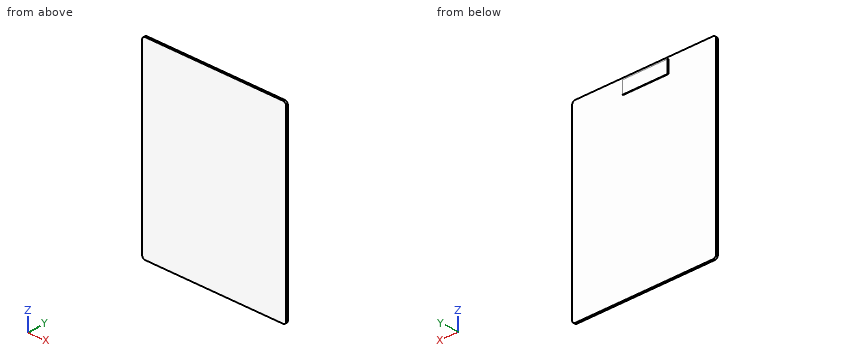
```python
from build123d import *

# Parameters (mm, degrees)
SKETCH1_W           = 230
SKETCH1_H           = 300
BOSS_EXTRUDE1_DEPTH = 3
FILLET1_R           = 5
SKETCH2_W           = 72.53015036
SKETCH2_H           = 20.073618637
BOSS_EXTRUDE2_DEPTH = 1


with BuildPart() as part:
    # Sketch1 → Boss-Extrude1 (new body)
    with BuildSketch(Plane(origin=(0, 0, 0), x_dir=(1, 0, 0), z_dir=(0, 1, 0))):
        with Locations((439.297793407, 824.401400972)):
            Rectangle(SKETCH1_W, SKETCH1_H)
    extrude(amount=BOSS_EXTRUDE1_DEPTH)

    # Fillet1
    fillet1_edges = [part.edges().sort_by_distance(p)[0] for p in [
        (554.297793407, 1.5, -674.401400972),
        (324.297793407, 1.5, -674.401400972),
        (324.297793407, 1.5, -974.401400972),
        (554.297793407, 1.5, -974.401400972),
    ]]
    fillet(fillet1_edges, radius=FILLET1_R)

    # Sketch2 → Boss-Extrude2 (add)
    with BuildSketch(Plane(origin=(0, 3, 0), x_dir=(1, 0, 0), z_dir=(0, 1, 0))):
        with Locations((436.94953533, 687.595411645)):
            Rectangle(SKETCH2_W, SKETCH2_H)
    extrude(amount=BOSS_EXTRUDE2_DEPTH)


solid = part.part
```
Work out the finished part from the listing and answer in its coordinate system (mm). Coordinates: 2 decimals unless noted, no trailing zeros. Order: outer loops, then holes, each group sorted by start corner. A loop starts at its lowest first (then second) coordinate and runs counter-clockwise, first axis right, second up. Notation, with made-up numbers: M 80,46 L 85,46 A21 cw 85,51 Z; hole C 76.25,34 d9. An arc over 180 degrees is marked long. Use CSV: the item, a comma, the result in double quotes.
1) Flat-ended cylindrical pins translate along their axes: pin 1 Ø2 at (x, z) = (470.5, -857.5) entering from +Y; pin 2 Ø0.8 at (y, z) = (3.5, -689) entering from -X; pin 3 Ø0.8 at (x, y) = (419, 3.5) entering from -Z. Find the tip coordinate at first contact, or state that the pin passes through.
Worked out:
pin 1,"stops at y = 3"
pin 2,"stops at x = 400.68"
pin 3,"stops at z = -697.63"
2) Consider line 1 (Z direction, x = 435, y = 3.8); line 2 (Y direction, x = 491.5, z = -725). Determine where each line is inside the solid, lowest interval first. Write a range as [from, to].
Worked out:
line 1,"z = [-697.63, -677.56]"
line 2,"y = [0, 3]"
3) Section A-A on x = 413 is taken. Write down the section's boundary in (y, z), plus the area to 3 significant figures.
Worked out:
outline,"M 0,-974.4 L 3,-974.4 L 3,-697.63 L 4,-697.63 L 4,-677.56 L 3,-677.56 L 3,-674.4 L 0,-674.4 Z"
area,"920 mm^2"
4) Section C-C on x = 344 is taken. Write down the section's boundary in (y, z).
Worked out:
outline,"M 0,-974.4 L 3,-974.4 L 3,-674.4 L 0,-674.4 Z"
5) Section B-B on z = -752 is taken. Write down the section's boundary in (x, y).
Worked out:
outline,"M 324.3,0 L 554.3,0 L 554.3,3 L 324.3,3 Z"
